Geometry check sheet. Reference: the model listing, model coordinates, mm. Face numbers are marked on the shaded views. A direction names the side the tool comes from. Round coordinates to 2 decimals unless told otherwise and drop trailing zeros. Order: outer loops, then holes, each group sorted by start corner. A loop starts at its lowest first (then second) coordinate and runs counter-clockwise, first axis right, second up. Notation, with made-up numbers: (22, 12.25) - (69, 12.25) arc R23 cw to (69, 21.25) - close; hole circle Ø3 at (26, 67). An arc over 180 degrees is marked (long way). Return JSON: item names as keys, results as strings. Group by question number.
Q1. Sectioned sample at A-A, the plane y = 0. Record the cut outline in (x, z), then the cut area to 3 significant figures.
Q2. Material ranges on line 1 along X through (y, z) = (33, 50); line 2 along Z through (x, y) = (132, -53.5); line 3 along Z through (x, y) = (103, 5.5), recorded low to high.
Q3. Draft check along X on the marked faces 6, 7 and 8. Enter one of: pulls with the +X half, pulls with the -X half, needs draft (parallel to the pull), parting line crosses it, or undercut.
Q4. Gauge pin test, flat ends, axial feed: pin 1 Ø12 at (y, z) = (-50.5, 20.5) entering from +X; pin 2 Ø10.5 at (x, y) = (102, 31) entering from -Z; pin 3 Ø1.5 at (x, y) = (164, 23) entering from +Z. Record the tip position at first contact, or that the pin passes through.
Q5. Sectioned sample at D-D, the plane x = 68. Record the cut outline in (y, z).
Q6. Tool access check on the marked faces 1, 2, 3, 4 and 5. Record the directions out of +Z, -Z, +X, -X, +Y, -Y that give a thin tool (end or side, any length) a straight path to the whole face; none if there is none.
Q7. Sectioned sample at B-B, the plane x = 99. Record the cut outline in (y, z).
Q8. Sectioned sample at C-C, the plane x = 27. Record the cut outline in (y, z).
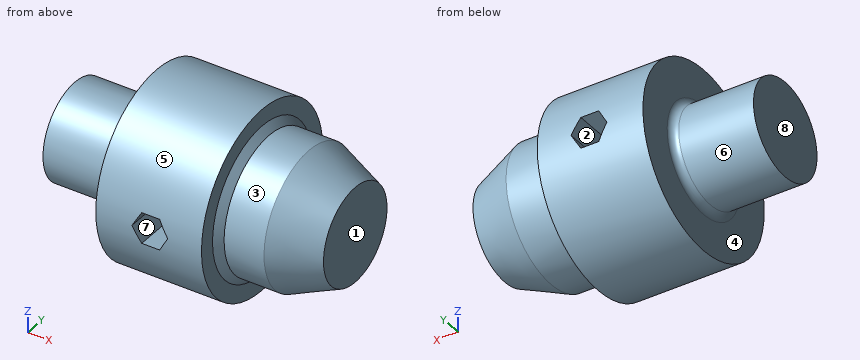
```python
from build123d import *

# Parameters (mm, degrees)
F2_R          = 5.08
F3_SIZE       = 5.08
F5_DEPTH      = 67.8453350663
F5_DEPTH_BACK = 67.8453350663


with BuildPart() as f1:
    # F0 (on Front) → F1 (revolve)
    with BuildSketch(Plane.XZ):
        Polygon((0, 35.0362285972), (0, 0), (205.1634937525, 0), (205.1634937525, 35.0362285972), (171.3081896305, 49.5771542192), (137.0425224304, 49.5771542192), (137.0425224304, 66.8453350663), (59.7526952624, 66.8453350663), (59.7526952624, 35.0362285972), align=None)
    revolve(axis=Axis((102.5817468762, 0, 0), (-1, 0, 0)))

    # F2
    f2_edges = [f1.edges().sort_by_distance(p)[0] for p in [
        (59.752695, 0, -35.036229),
    ]]
    fillet(f2_edges, radius=F2_R)

    # F3
    f3_edges = [f1.edges().sort_by_distance(p)[0] for p in [
        (137.042522, 0, -49.577154),
    ]]
    chamfer(f3_edges, length=F3_SIZE)

    # F4 (on Front) → F5 (cut, two sides)
    with BuildSketch(Plane.XZ) as f5_sk:
        Polygon((92.6886847283, -11.3443676382), (105.7880321477, -11.3443676382), (112.3377058575, 0), (105.7880321477, 11.3443676382), (92.6886847283, 11.3443676382), (86.1390110186, 0), align=None)
    extrude(amount=F5_DEPTH, mode=Mode.SUBTRACT)
    extrude(f5_sk.sketch, amount=-F5_DEPTH_BACK, mode=Mode.SUBTRACT)


solid = f1.part
```
Reply:
{
 "1": {"outline": "(0, -35.04) - (54.67, -35.04) arc R5.08 cw to (59.75, -40.12) - (59.75, -66.85) - (137.04, -66.85) - (137.04, -54.66) - (142.12, -49.58) - (171.31, -49.58) - (205.16, -35.04) - (205.16, 35.04) - (171.31, 49.58) - (142.12, 49.58) - (137.04, 54.66) - (137.04, 66.85) - (59.75, 66.85) - (59.75, 40.12) arc R5.08 cw to (54.67, 35.04) - (0, 35.04) - close; hole (86.14, 0) - (92.69, -11.34) - (105.79, -11.34) - (112.34, 0) - (105.79, 11.34) - (92.69, 11.34) - close", "area": "20,400 mm^2"},
 "2": {"line 1": "59.75 to 137.04", "line 2": "-40.08 to 40.08", "line 3": "-66.62 to -11.34, 11.34 to 66.62"},
 "3": {"face 6": "needs draft", "face 7": "undercut", "face 8": "pulls with the -X half"},
 "4": {"pin 1": "x = 173.81", "pin 2": "z = -61.69", "pin 3": "z = 44.3"},
 "5": {"outline": "circle Ø133.69 at (0, 0)"},
 "6": {"face 1": "+Z, -Z, +X, +Y, -Y", "face 2": "+Y, -Y", "face 3": "+X", "face 4": "-X", "face 5": "+X, -X"},
 "7": {"outline": "(-65.88, -11.34) arc R66.85 ccw to (65.88, -11.34) - close; (-65.88, 11.34) - (65.88, 11.34) arc R66.85 ccw to start"},
 "8": {"outline": "circle Ø70.07 at (0, 0)"}
}
